Design review of the part shown in the three views and the two pictorial views. Dimensions are in mm from the part's minimum x, y and z. Coordinates: 2 decimals unless noted, no trailing zeros. Write each loop counter-clockwise with the first axis right and the second up, starting at its lowest first coordinate (ties: lowest second). Pieces come first, ordered by that corner, then holes. Notation, with made-up numbers: (55, -14) -> (62, -14) arc R26 ccw to (62, 22) -> close; hole circle Ø7 at (-13.75, -5). An arc over 180 degrees is marked (long way). Answer in a Markdown table with one row per item. Add a question column.
Item 1: Clearance check with flat-ended pins moving along their axes: P1, Ø12, axis at x = 7.5, z = 24.5, coming from the +Y side; P2, Ø1.5, axis at y = 14, z = 18, coming from the +X side; P3, Ø8, axis at x = 6, y = 7, coming from the -Z side. State where each tip first meets the part, or that it passes through.
Item 2: Take a section at B-B, the plane y = 12.75. Write out the cut boundary in (x, z), and give its area (3 significant figures).
Item 3: To check wall thickness, follow line 1 (X direction, y = 14.5, z = 6.5). State the ranges of the line that lie inside material, in increasing order.
Item 4: Take a section at A-A, the plane z = 25.5. Write out the cut boundary in (x, y).
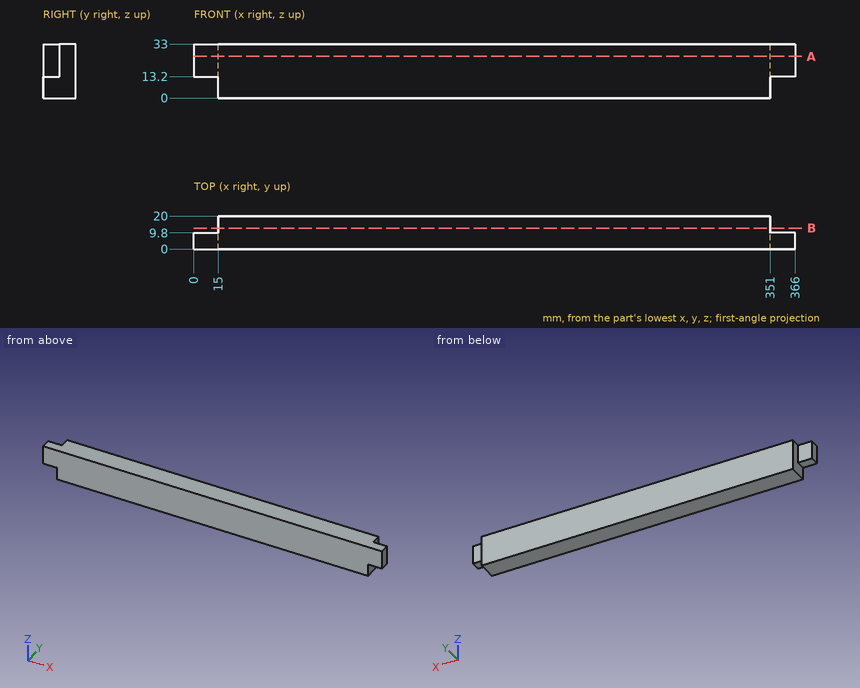
Answers:
| question | item | result |
|---|---|---|
| 1 | P1 | stops at y = 9.8 |
| 1 | P2 | stops at x = 351 |
| 1 | P3 | stops at z = 13.2 |
| 2 | outline | (15, 0) -> (351, 0) -> (351, 33) -> (15, 33) -> close |
| 2 | area | 11,100 mm^2 |
| 3 | line 1 | x = 15 to 351 |
| 4 | outline | (0, 0) -> (366, 0) -> (366, 9.8) -> (351, 9.8) -> (351, 20) -> (15, 20) -> (15, 9.8) -> (0, 9.8) -> close |
